```python
from build123d import *

# Parameters (mm, degrees)
F1_DEPTH  = 5.5
F2_DEPTH  = 9.5
F5_DEPTH  = 4
F7_DEPTH  = 4
F8_R      = 5
F9_R      = 5
F10_R     = 5
F11_R     = 5
F3_W      = 12.9391151695
F3_H      = 8
F12_DEPTH = 40


# Not quite as in the source:
# - a feature names something its author has since deleted; it is built from what else it names


with BuildPart() as f1:
    # F0 (on Top) → F1 (new body, symmetric)
    with BuildSketch(Plane.XY):
        Polygon((45.3994634662, -11.2350502836), (29.5210014421, -9.8458648622), (25.8999169252, -51.2350502836), (41.8999169252, -51.2350502836), align=None)
    extrude(amount=F1_DEPTH, both=True)

    # F0 (on Top) → F2 (join, symmetric)
    with BuildSketch(Plane.XY):
        Polygon((41.8999169252, -51.2350502836), (25.8999169252, -51.2350502836), (22.3999169252, -51.2350502836), (22.3999169252, -55.7350502836), (45.3999169252, -55.7350502836), (45.3999169252, -51.2350502836), align=None)
    extrude(amount=F2_DEPTH, both=True)

    # F4 (on face) → F5 (join)
    with BuildSketch(Plane.XY.offset(5.5)):
        with BuildLine():
            Line((29.8999169252, -51.2350502836), (37.8999169252, -51.2350502836))
            ThreePointArc((37.8999169252, -51.2350502836), (33.8999169252, -47.2350502836), (29.8999169252, -51.2350502836))
        make_face()
    extrude(amount=F5_DEPTH)

    # F6 (on face) → F7 (join)
    with BuildSketch(Plane(origin=(0, 0, -5.5), x_dir=(1, 0, 0), z_dir=(0, 0, -1))):
        with BuildLine():
            ThreePointArc((29.8999169252, 51.2350502836), (33.8999169252, 47.2350502836), (37.8999169252, 51.2350502836))
            Line((37.8999169252, 51.2350502836), (29.8999169252, 51.2350502836))
        make_face()
    extrude(amount=F7_DEPTH)

    # F8
    f8_edges = [f1.edges().sort_by_distance(p)[0] for p in [
        (22.399917, -53.48505, 9.5),
    ]]
    fillet(f8_edges, radius=F8_R)

    # F9
    f9_edges = [f1.edges().sort_by_distance(p)[0] for p in [
        (45.399917, -53.48505, 9.5),
    ]]
    fillet(f9_edges, radius=F9_R)

    # F10
    f10_edges = [f1.edges().sort_by_distance(p)[0] for p in [
        (45.399917, -53.48505, -9.5),
    ]]
    fillet(f10_edges, radius=F10_R)

    # F11
    f11_edges = [f1.edges().sort_by_distance(p)[0] for p in [
        (22.399917, -53.48505, -9.5),
    ]]
    fillet(f11_edges, radius=F11_R)

    # F3 (on face) → F12 (cut)
    with BuildSketch(Plane(origin=(-0.6306130728, -7.2079404052, 0), x_dir=(-0.9961946981, 0.0871557427, 0), z_dir=(0.0871557427, 0.9961946981, 0))):
        with Locations((-38.2363463688, 0)):
            Rectangle(F3_W, F3_H)
    extrude(amount=-F12_DEPTH, mode=Mode.SUBTRACT)


solid = f1.part
```
Design review of the part built by this model. Coordinates are the model's own, in mm. A direction names the side the tool comes from. Coordinates: 2 decimals unless noted, no trailing zeros. Loops run counter-clockwise (first coordinate to the right, second up) from the corner with the lowest first, then second, coordinate; pieces in that order, holes last. Notation, with made-up numbers: (24, 18) - (42, 18) arc R15 cw to (42, 29) - close; hole circle Ø11 at (25.25, 53). An arc over 180 degrees is marked (long way). Use CSV: the item, a comma, the result in double quotes. Start each with the question number.
1) Consider section A-A on z = -2.25. Write out the cut boundary in (x, y), then the cut area to 3 significant figures.
2) The part is to be moulded in two halves that separate along Z. For faces 4 (the flat face through (36, -30, -4)), 5 (the flat face through (22.4, -53, 0)), 6 (the cylindrical face through (23.9, -53.52, -8.07)), 7 (the cylindrical face through (23.83, -53.52, 8)), say which applies: +Z half, -Z half, draft (parallel to the pull), parting line (faces both ways), or undercut.
3) Consider section C-C on y = -22. Write out the cut boundary in (x, z), then the cut area to 3 significant figures.
4) For pin 1 Ø1 at (x, y) = (33.5, -38) entering from -Z; pin 2 Ø6 at (x, y) = (31.5, -40.5) entering from +Z; pin 3 Ø1 at (x, z) = (32.5, 0.5) entering from +Y, all flat-tipped, find the tip position at first contact; note any pin that passes through.
5) Consider section B-B on x = 41.25. Write out the cut boundary in (y, z).
6) Consider section D-D on z = -6. Write out the cut boundary in (x, y), then the cut area to 3 significant figures.
7) Wall thickness on L1, parallel to Z at x = 38.5, y = -28; L2, parallel to Z at x = 42, y = -38.5; L3, parallel to X at y = -33, z = -2.5: over which ranges is each line inside the solid? List them lowest first. Write a range as from..to.
8) Tool access review of faces 1 (the flat face through (34.1, -50.4, 0.1)), 2 (the flat face through (43, -51.235, 0)), 3 (the cylindrical face through (33.988, -47.236, 7.472)): name each direction out of +Z, -Z, +X, -X, +Y, -Y from which nothing blocks a thin tool from reaching the whole face with its end or side.
Geometry says:
1,outline,"(22.4, -55.74) - (45.4, -55.74) - (45.4, -51.24) - (41.9, -51.24) - (45.4, -11.24) - (43.91, -11.1) - (40.42, -50.95) - (27.53, -49.82) - (31.02, -9.98) - (29.52, -9.85) - (25.9, -51.24) - (22.4, -51.24) - close"
1,area,"237 mm^2"
2,face 4,"undercut"
2,face 5,"draft"
2,face 6,"-Z half"
2,face 7,"+Z half"
3,outline,"(28.46, -5.5) - (44.46, -5.5) - (44.46, 5.5) - (28.46, 5.5) - close; hole (29.96, -4) - (42.95, -4) - (42.95, 4) - (29.96, 4) - close"
3,area,"72.1 mm^2"
4,pin 1,"z = -5.5"
4,pin 2,"z = 5.5"
4,pin 3,"y = -50.22"
5,outline,"(-55.74, -9.43) - (-51.24, -9.43) - (-51.24, -5.5) - (-10.87, -5.5) - (-10.87, -4) - (-41.45, -4) - (-41.45, 4) - (-10.87, 4) - (-10.87, 5.5) - (-51.24, 5.5) - (-51.24, 9.43) - (-55.74, 9.43) - close"
6,outline,"(22.63, -55.74) - (45.17, -55.74) - (45.17, -51.24) - (37.9, -51.24) arc R4 ccw to (29.9, -51.24) - (22.63, -51.24) - close"
6,area,"127 mm^2"
7,L1,"-5.5..-4, 4..5.5"
7,L2,"-5.5..5.5"
7,L3,"27.5..29, 41.99..43.5"
8,face 1,"none"
8,face 2,"+X"
8,face 3,"+Z, +Y"
